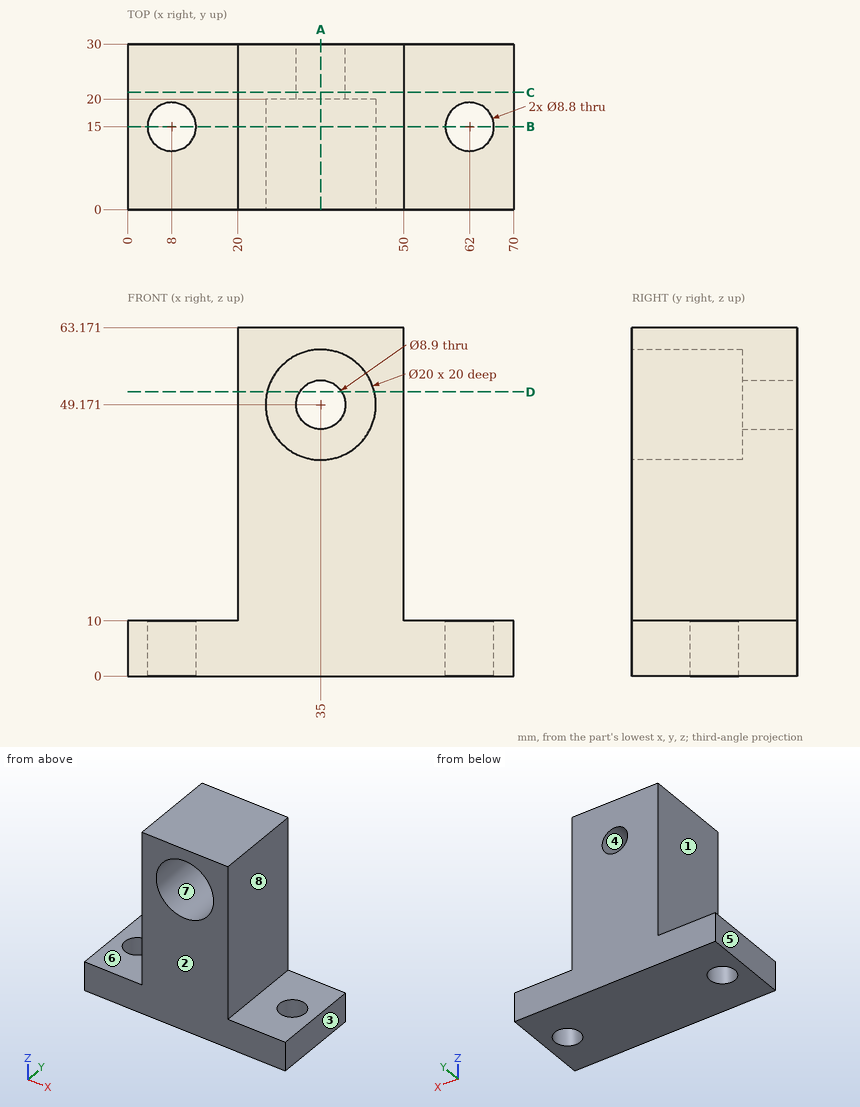
Answer from the drawing. Dimensions are ordinates in mm from the lowest x, y and z of the part. A direction names the side the tool comes from. Coordinates: 2 decimals unless noted, no trailing zeros. Write each loop counter-clockwise with the first axis right and the second up, starting at its lowest first coordinate (ties: lowest second). Pieces come first, ordered by that corner, then holes. Notation, with made-up numbers: (65, 51.5) - (72, 51.5) arc R11 cw to (72, 58.5) - close; hole circle Ø2 at (58, 77). An arc over 180 degrees is marked (long way). Return JSON: item names as keys, results as strings. Group by question number.
Q1. The part is cut by section D-D on z = 51.5. Write down the section's boundary in (x, y) (1 decimal), and give its area (3 significant figures).
Q2. The part is cut by section A-A on x = 35. Write down the section's boundary in (y, z).
Q3. Which of the six approach directions +Z, -Z, +X, -X, +Y, -Y give full straight-line access (tool end or side, diameter ignored) to the marked faces 5, 6, 7 and 8?
Q4. The part is cut by section C-C on y = 21.25. Write down the section's boundary in (x, z).
Q5. The part is cut by section B-B on y = 15. Write down the section's boundary in (x, z).
Q6. For a pull along X with two mould halves and no side action, classify the marked faces 1, 2, 3 and 4 as +X half, -X half, draft (parallel to the pull), parting line (faces both ways), or undercut.
Q7. Flat-ended cylindrical pins translate along their axes: pin 1 Ø23 at (x, z) = (35, 49.17) entering from +Y; pin 2 Ø6 at (x, y) = (6.5, 17) entering from +Z; pin 3 Ø15 at (y, z) = (18.5, 40) entering from -X; pin 4 Ø10 at (y, z) = (3.5, 35) entering from +X. Find the tip coordinate at first contact, or state that the pin passes through.
Q8. Find the intervals of material crossed by line 1 along Z through (x, y) = (35, 26); line 2 along Y through (x, z) = (62, 4.5); line 3 along Z through (x, y) = (35, 12.5), in increasing order. Write a range as [from, to].
Evaluation:
{
 "1": {"outline": "(20, 0) - (25.3, 0) - (25.3, 20) - (31.2, 20) - (31.2, 30) - (20, 30) - close; (38.8, 20) - (44.7, 20) - (44.7, 0) - (50, 0) - (50, 30) - (38.8, 30) - close", "area": "435 mm2"},
 "2": {"outline": "(0, 0) - (30, 0) - (30, 44.72) - (20, 44.72) - (20, 39.17) - (0, 39.17) - close; (0, 59.17) - (20, 59.17) - (20, 53.62) - (30, 53.62) - (30, 63.17) - (0, 63.17) - close"},
 "3": {"face 5": "+Z, -Z, -X, +Y, -Y", "face 6": "+Z, -X, +Y, -Y", "face 7": "-Y", "face 8": "+Z, +X, +Y, -Y"},
 "4": {"outline": "(0, 0) - (70, 0) - (70, 10) - (50, 10) - (50, 63.17) - (20, 63.17) - (20, 10) - (0, 10) - close; hole circle Ø8.9 at (35, 49.17)"},
 "5": {"outline": "(0, 0) - (3.6, 0) - (3.6, 10) - (0, 10) - close; (12.4, 0) - (57.6, 0) - (57.6, 10) - (50, 10) - (50, 63.17) - (20, 63.17) - (20, 10) - (12.4, 10) - close; (66.4, 0) - (70, 0) - (70, 10) - (66.4, 10) - close; hole circle Ø20 at (35, 49.17)"},
 "6": {"face 1": "-X half", "face 2": "draft", "face 3": "+X half", "face 4": "undercut"},
 "7": {"pin 1": "stops at y = 30", "pin 2": "stops at z = 10", "pin 3": "stops at x = 20", "pin 4": "stops at x = 50"},
 "8": {"line 1": "z = [0, 44.72], [53.62, 63.17]", "line 2": "y = [0, 10.6], [19.4, 30]", "line 3": "z = [0, 39.17], [59.17, 63.17]"}
}
